```python
from build123d import *

# Parameters (mm, degrees)
SKETCH1_R                 = 18.5
BOSS_EXTRUDE1_DEPTH       = 30
SKETCH2_R                 = 18.1
BOSS_EXTRUDE2_DEPTH       = 33.3
SKETCH3_R                 = 6
BOSS_EXTRUDE3_DEPTH       = 5
SKETCH4_R                 = 3
BOSS_EXTRUDE4_DEPTH       = 1
BOSS_EXTRUDE5_DEPTH       = 14
M3X0_5_TAPPED_HOLE1_D     = 2.5
M3X0_5_TAPPED_HOLE1_DEPTH = 6
M3X0_5_TAPPED_HOLE1_TIP   = 0.751075774


with BuildPart() as part:
    # Sketch1 → Boss-Extrude1 (new body)
    with BuildSketch(Plane.XY):
        Circle(SKETCH1_R)
    extrude(amount=BOSS_EXTRUDE1_DEPTH)

    # Sketch2 → Boss-Extrude2 (add)
    with BuildSketch(Plane(origin=(0, 0, 0), x_dir=(-1, 0, 0), z_dir=(0, 0, -1))):
        Circle(SKETCH2_R)
    extrude(amount=BOSS_EXTRUDE2_DEPTH)

    # Sketch3 → Boss-Extrude3 (add)
    with BuildSketch(Plane.XY.offset(30)):
        Circle(SKETCH3_R)
    extrude(amount=BOSS_EXTRUDE3_DEPTH)

    # Sketch4 → Boss-Extrude4 (add)
    with BuildSketch(Plane.XY.offset(35)):
        Circle(SKETCH4_R)
    extrude(amount=BOSS_EXTRUDE4_DEPTH)

    # Sketch5 → Boss-Extrude5 (add)
    with BuildSketch(Plane.XY.offset(36)):
        with BuildLine():
            Line((-1.658312395, 2.5), (1.658312395, 2.5))
            ThreePointArc((1.658312395, 2.5), (0, -3), (-1.658312395, 2.5))
        make_face()
    extrude(amount=BOSS_EXTRUDE5_DEPTH)

    # M3x0.5 Tapped Hole1
    with Locations(Plane.XY.offset(30)):
        with Locations((0, 15.5), (13.423393759, 7.75), (13.423393759, -7.75), (0, -15.5), (-13.423393759, -7.75), (-13.423393759, 7.75)):
            Hole(M3X0_5_TAPPED_HOLE1_D / 2, depth=M3X0_5_TAPPED_HOLE1_DEPTH)
            with Locations((0, 0, -(M3X0_5_TAPPED_HOLE1_DEPTH + M3X0_5_TAPPED_HOLE1_TIP / 2))):  # 118° drill point
                Cone(0, M3X0_5_TAPPED_HOLE1_D / 2, M3X0_5_TAPPED_HOLE1_TIP, mode=Mode.SUBTRACT)


solid = part.part
```
Could you check a few things on this model? Use its own coordinates, in mm. A direction names the side the tool comes from. Give positions to 0.01 mm unless a question says otherwise; leave off trailing zeros. Order: outer loops, then holes, each group sorted by start corner. A loop starts at its lowest first (then second) coordinate and runs counter-clockwise, first axis right, second up.
Q1. We'd pull the mould along Y, two halves only. Please class faces 4 (the flat face through (0, 0, 50)), 5 (the cylindrical face through (12.27, 7.27, 26.96)), 6 (the cylindrical face through (-4.01, -18.06, 14.79)): +Y half, -Y half, draft (parallel to the pull), parting line (faces both ways), or undercut.
Q2. If I drill on line 1 along Y through (x, z) = (0, 26.3); line 2 along Z through (x, y) = (1, 11.5); line 3 along X through (y, z) = (7.75, 26.7), over which ranges is the centre line in solid material (lowest first)?
Q3. I'm going to push flat-ended pins straight in: P1, Ø1.5, axis at x = 13.42, y = -7.75, coming from the +Z side; P2, Ø6, axis at x = -7, z = 7, coming from the +Y side; P3, Ø5, axis at x = -10.5, y = -2.5, coming from the +Z side. Where does each tip first touch, or does it pass through?
Q4. Suppose I cut it at B-B, the plane y = 0. Write out the boundary of the cut face in (x, z), and give its area (3 significant figures).
Q5. For faces 1 (the cylindrical face through (-0.672, 16.554, 26.958)), 2 (the flat face through (13.6, -12.2, 0)), 3 (the flat face through (0, 2.5, 43)), which set-ups out of +Z, -Z, +X, -X, +Y, -Y let a thin tool reach every point of the face, with its end or its side?
Q6. Suppose I cut it at C-C, the plane z = -1. Write out the boundary of the cut face in (x, y).
Q7. Suppose I cut it at D-D, the plane y = -12. Write out the boundary of the cut face in (x, z).
Q8. Suppose I cut it at A-A, the plane x = 10. Write out the boundary of the cut face in (y, z).
Solution:
1. face 4: draft
1. face 5: undercut
1. face 6: parting line
2. line 1: y = -18.5 to -16.75, -14.25 to 14.25, 16.75 to 18.5
2. line 2: z = -33.3 to 30
2. line 3: x = -16.8 to -14.67, -12.17 to 12.17, 14.67 to 16.8
3. P1: stops at z = 23.7
3. P2: stops at y = 18.06
3. P3: stops at z = 30
4. outline: (-18.5, 0) - (-18.1, 0) - (-18.1, -33.3) - (18.1, -33.3) - (18.1, 0) - (18.5, 0) - (18.5, 30) - (6, 30) - (6, 35) - (3, 35) - (3, 50) - (-3, 50) - (-3, 35) - (-6, 35) - (-6, 30) - (-18.5, 30) - close
4. area: 2,470 mm2
5. face 1: +Z
5. face 2: -Z
5. face 3: +Z, +X, -X, +Y
6. outline: circle Ø36.2 at (0, 0)
7. outline: (-14.08, 0) - (-13.55, 0) - (-13.55, -33.3) - (13.55, -33.3) - (13.55, 0) - (14.08, 0) - (14.08, 30) - (-14.08, 30) - close
8. outline: (-15.56, 0) - (-15.09, 0) - (-15.09, -33.3) - (15.09, -33.3) - (15.09, 0) - (15.56, 0) - (15.56, 30) - (-15.56, 30) - close
